Model file for the job. Use its own axes, mm. A direction names the side the tool comes from. Coordinates: 2 decimals unless noted, no trailing zeros. Loops run counter-clockwise (first coordinate to the right, second up) from the corner with the lowest first, then second, coordinate; pieces in that order, holes last.
from build123d import *

# Parameters (mm, degrees)
F0_W     = 45
F0_H     = 45
F1_DEPTH = 1.0414
F2_DEPTH = 4.6736
F4_DEPTH = 0.254


with BuildPart() as f1:
    # F0 (on Front) → F1 (new body)
    with BuildSketch(Plane.XZ):
        with Locations((-95.2571389369, 31.5730149047)):
            Rectangle(F0_W, F0_H)
        with BuildLine():
            ThreePointArc((-114.7571389369, 49.4855149047), (-115.879670952, 52.1955469198), (-113.1696389369, 51.0730149047))
            Line((-113.1696389369, 51.0730149047), (-77.3446389369, 51.0730149047))
            ThreePointArc((-77.3446389369, 51.0730149047), (-75.7571389369, 52.6605149047), (-74.1696389369, 51.0730149047))
            ThreePointArc((-74.1696389369, 51.0730149047), (-74.6346069217, 49.9504828895), (-75.7571389369, 49.4855149047))
            Line((-75.7571389369, 49.4855149047), (-75.7571389369, 48.7390149047))
            Line((-75.7571389369, 48.7390149047), (-75.3987389369, 48.7390149047))
            Line((-75.3987389369, 48.7390149047), (-75.3987389369, 14.7030149047))
            Line((-75.3987389369, 14.7030149047), (-75.7571389369, 14.7030149047))
            Line((-75.7571389369, 14.7030149047), (-75.7571389369, 13.6605149047))
            ThreePointArc((-75.7571389369, 13.6605149047), (-74.6346069217, 13.1955469198), (-74.1696389369, 12.0730149047))
            ThreePointArc((-74.1696389369, 12.0730149047), (-75.7571389369, 10.4855149047), (-77.3446389369, 12.0730149047))
            Line((-77.3446389369, 12.0730149047), (-113.1696389369, 12.0730149047))
            ThreePointArc((-113.1696389369, 12.0730149047), (-115.879670952, 10.9504828895), (-114.7571389369, 13.6605149047))
            Line((-114.7571389369, 13.6605149047), (-114.7571389369, 14.7030149047))
            Line((-114.7571389369, 14.7030149047), (-115.1155389369, 14.7030149047))
            Line((-115.1155389369, 14.7030149047), (-115.1155389369, 48.7390149047))
            Line((-115.1155389369, 48.7390149047), (-114.7571389369, 48.7390149047))
            Line((-114.7571389369, 48.7390149047), (-114.7571389369, 49.4855149047))
        make_face(mode=Mode.SUBTRACT)
        with BuildLine():
            Line((-77.3446389369, 51.0730149047), (-113.1696389369, 51.0730149047))
            ThreePointArc((-113.1696389369, 51.0730149047), (-113.6346069217, 49.9504828895), (-114.7571389369, 49.4855149047))
            Line((-114.7571389369, 49.4855149047), (-114.7571389369, 48.7390149047))
            Line((-114.7571389369, 48.7390149047), (-75.7571389369, 48.7390149047))
            Line((-75.7571389369, 48.7390149047), (-75.7571389369, 49.4855149047))
            ThreePointArc((-75.7571389369, 49.4855149047), (-76.879670952, 49.9504828895), (-77.3446389369, 51.0730149047))
        make_face()
        with BuildLine():
            Line((-75.7571389369, 14.7030149047), (-114.7571389369, 14.7030149047))
            Line((-114.7571389369, 14.7030149047), (-114.7571389369, 13.6605149047))
            ThreePointArc((-114.7571389369, 13.6605149047), (-113.6346069217, 13.1955469198), (-113.1696389369, 12.0730149047))
            Line((-113.1696389369, 12.0730149047), (-77.3446389369, 12.0730149047))
            ThreePointArc((-77.3446389369, 12.0730149047), (-76.879670952, 13.1955469198), (-75.7571389369, 13.6605149047))
            Line((-75.7571389369, 13.6605149047), (-75.7571389369, 14.7030149047))
        make_face()
    extrude(amount=F1_DEPTH)

    # F0 (on Front) → F2 (join)
    with BuildSketch(Plane.XZ):
        Polygon((-75.7571389369, 48.7390149047), (-114.7571389369, 48.7390149047), (-115.1155389369, 48.7390149047), (-115.1155389369, 14.7030149047), (-114.7571389369, 14.7030149047), (-75.7571389369, 14.7030149047), (-75.3987389369, 14.7030149047), (-75.3987389369, 48.7390149047), align=None)
    extrude(amount=F2_DEPTH)

    # F3 (on face) → F4 (cut)
    with BuildSketch(Plane.XZ.offset(4.6736)):
        with BuildLine():
            Line((-78.5737389369, 47.3420149047), (-111.9405389369, 47.3420149047))
            ThreePointArc((-111.9405389369, 47.3420149047), (-113.1977747938, 46.8212507616), (-113.7185389369, 45.5640149047))
            Line((-113.7185389369, 45.5640149047), (-113.7185389369, 24.5582149047))
            ThreePointArc((-113.7185389369, 24.5582149047), (-113.1977747938, 23.3009790477), (-111.9405389369, 22.7802149047))
            Line((-111.9405389369, 22.7802149047), (-78.5737389369, 22.7802149047))
            ThreePointArc((-78.5737389369, 22.7802149047), (-77.3165030799, 23.3009790477), (-76.7957389369, 24.5582149047))
            Line((-76.7957389369, 24.5582149047), (-76.7957389369, 45.5640149047))
            ThreePointArc((-76.7957389369, 45.5640149047), (-77.3165030799, 46.8212507616), (-78.5737389369, 47.3420149047))
        make_face()
    extrude(amount=-F4_DEPTH, mode=Mode.SUBTRACT)


solid = f1.part
Q1. Which spindle directions (+Z, -Z, +X, -X, +Y, -Y) get a long thin tool onto all of the face, cutting with end or side? Do faces 1 (the flat face through (-95, -3, 48.739)), 2 (the flat face through (-94, -4.674, 22)), 3 (the flat face through (-75.399, -3, 31)), 4 (the flat face through (-115.116, -3, 32)), 5 (the flat face through (-72.757, -0.5, 31.3)). Say none if no direction does.
Answers:
face 1: +Z, +X, -X, -Y
face 2: +Z, -Z, +X, -X, -Y
face 3: +Z, -Z, +X, -Y
face 4: +Z, -Z, -X, -Y
face 5: +Z, -Z, +X, +Y, -Y
Q2. Drill centre lines: line 1 (X direction, y = -3.85, z = 39.5); line 2 (Y direction, x = -82, z = 13); line 3 (Z direction, x = -107.5, y = -3.6). Where is each one in solid material? Low to high.
Answers:
line 1: x = -115.12 to -75.4
line 2: y = -1.04 to 0
line 3: z = 14.7 to 48.74
Q3. Flat gauge pins, fed straight in: P1, Ø5, axis at x = -95.5, z = 36, coming from the -Y side; P2, Ø1.9, axis at x = -114.76, z = 12.07, coming from the -Y side; P3, Ø1.8, axis at y = -3, z = 32.5, coming from the +X side; P4, Ø1.1, axis at y = -3.5, z = 35, coming from the -X side. Where does each tip first touch, or does it go through?
Answers:
P1: stops at y = -4.42
P2: passes through
P3: stops at x = -75.4
P4: stops at x = -115.12
Q4. Slice it at B-B (x = -85). List the corners of the cut face in (y, z).
Answers:
outline: (-4.67, 14.7) - (-1.04, 14.7) - (-1.04, 9.07) - (0, 9.07) - (0, 54.07) - (-1.04, 54.07) - (-1.04, 48.74) - (-4.67, 48.74) - (-4.67, 47.34) - (-4.42, 47.34) - (-4.42, 22.78) - (-4.67, 22.78) - close
Q5. Slice it at C-C (y = -1.7). List the corners of the cut face in (x, z).
Answers:
outline: (-115.12, 14.7) - (-75.4, 14.7) - (-75.4, 48.74) - (-115.12, 48.74) - close
Q6. Slice it at D-D (z = 40.5). List the corners of the cut face in (x, y).
Answers:
outline: (-117.76, -1.04) - (-115.12, -1.04) - (-115.12, -4.67) - (-113.72, -4.67) - (-113.72, -4.42) - (-76.8, -4.42) - (-76.8, -4.67) - (-75.4, -4.67) - (-75.4, -1.04) - (-72.76, -1.04) - (-72.76, 0) - (-117.76, 0) - close
Q7. Mould opens along Z. For faces 6 (the flat face through (-96, -4.42, 35)), 7 (the flat face through (-96, 0, 32)), 8 (the flat face through (-95.6, -0.5, 54.073)), 9 (the flat face through (-96, -3, 14.703)) say: +Z half, -Z half, draft (parallel to the pull), parting line (faces both ways), or undercut.
Answers:
face 6: undercut
face 7: draft
face 8: +Z half
face 9: -Z half
Q8. Slice it at A-A (z = 19.5). List the corners of the cut face in (x, y).
Answers:
outline: (-117.76, -1.04) - (-115.12, -1.04) - (-115.12, -4.67) - (-75.4, -4.67) - (-75.4, -1.04) - (-72.76, -1.04) - (-72.76, 0) - (-117.76, 0) - close
